from build123d import *

# Parameters (mm, degrees)
BOSS_EXTRUDE1_DEPTH = 12.7
SKETCH3_R           = 2.286
CUT_EXTRUDE1_DEPTH  = 232.948038146
CAVITY1_START       = -1
CAVITY1_OUTLINE_R   = 2.286
CAVITY1_DEPTH       = 15
CUT_EXTRUDE2_DEPTH  = 232.948038146
FILLET1_R           = 12.7
FILLET2_R           = 2.54
FILLET3_R           = 20.32
FILLET4_R           = 17.78
SKETCH5_W           = 16.51
SKETCH5_H           = 5.08
CUT_EXTRUDE3_DEPTH  = 230.304470216
FILLET5_R           = 127
FILLET6_R           = 50.8


with BuildPart() as part:
    # Sketch1 → Boss-Extrude1 (new body)
    with BuildSketch(Plane(origin=(0, 0, 0), x_dir=(1, 0, 0), z_dir=(0, 1, 0))):
        with BuildLine():
            Line((0, 0), (38.1, 0))
            Line((38.1, 0), (38.1, 25.4))
            ThreePointArc((38.1, 25.4), (19.393233119, 60.430202712), (-12.7, 83.82))
            Line((-12.7, 83.82), (-165.1, 83.82))
            ThreePointArc((-165.1, 83.82), (-197.193233119, 60.430202712), (-215.9, 25.4))
            Line((-215.9, 25.4), (-215.9, 0))
            Line((-215.9, 0), (-177.8, 0))
            ThreePointArc((-177.8, 0), (-166.58502935, 42.017514675), (-139.7, 76.2))
            Line((-139.7, 76.2), (-38.1, 76.2))
            ThreePointArc((-38.1, 76.2), (-11.21497065, 42.017514675), (0, 0))
        make_face()
    extrude(amount=BOSS_EXTRUDE1_DEPTH)

    # Sketch3 → Cut-Extrude1 (cut, through all)
    with BuildSketch(Plane(origin=(0, 12.7, 0), x_dir=(1, 0, 0), z_dir=(0, 1, 0))):
        with Locations(Location((19.05, 28.956, 0), (0, 0, 270))):
            Circle(SKETCH3_R)
    extrude(amount=-CUT_EXTRUDE1_DEPTH, mode=Mode.SUBTRACT)

    # Cavity1: read off the stored shape, not the designer's step
    # Cavity1 outline → Cavity1 (cut)
    with BuildSketch(Plane(origin=(0, 0, 0), x_dir=(1, 0, 0), z_dir=(0, 1, 0)).offset(CAVITY1_START)):
        with BuildLine():
            ThreePointArc((13.557199982, 23.797473427), (13.721594677, 23.627834729), (13.891225968, 23.463432392))
            ThreePointArc((13.891225968, 23.463432392), (15.144839416, 23.828362371), (16.075009031, 24.744607454))
            ThreePointArc((16.075009031, 24.744607454), (16.471799412, 24.490657889), (16.890111616, 24.273983275))
            ThreePointArc((16.890111616, 24.273983275), (16.561647975, 23.010325013), (16.872358933, 21.742184932))
            ThreePointArc((16.872358933, 21.742184932), (17.099548264, 21.677470858), (17.32865444, 21.619909903))
            ThreePointArc((17.32865444, 21.619909903), (18.231850543, 22.56275526), (18.579278518, 23.821331586))
            ThreePointArc((18.579278518, 23.821331586), (19.049883851, 23.799800001), (19.520490153, 23.821310384))
            ThreePointArc((19.520490153, 23.821310384), (19.867861426, 22.562718407), (20.77101505, 21.61983236))
            ThreePointArc((20.77101505, 21.61983236), (21.000123819, 21.677382993), (21.227316065, 21.742086832))
            ThreePointArc((21.227316065, 21.742086832), (21.538084156, 23.010212914), (21.209677446, 24.273885972))
            ThreePointArc((21.209677446, 24.273885972), (21.627999411, 24.490541739), (22.024801233, 24.744473428))
            ThreePointArc((22.024801233, 24.744473428), (22.954929568, 23.828186439), (24.208526573, 23.463199982))
            ThreePointArc((24.208526573, 23.463199982), (24.378165271, 23.627594677), (24.542567608, 23.797225968))
            ThreePointArc((24.542567608, 23.797225968), (24.177637629, 25.050839416), (23.261392546, 25.981009031))
            ThreePointArc((23.261392546, 25.981009031), (23.515342111, 26.377799412), (23.732016725, 26.796111616))
            ThreePointArc((23.732016725, 26.796111616), (24.995674987, 26.467647975), (26.263815068, 26.778358933))
            ThreePointArc((26.263815068, 26.778358933), (26.328529142, 27.005548264), (26.386090097, 27.23465444))
            ThreePointArc((26.386090097, 27.23465444), (25.44324474, 28.137850543), (24.184668414, 28.485278518))
            ThreePointArc((24.184668414, 28.485278518), (24.206199999, 28.955883851), (24.184689616, 29.426490153))
            ThreePointArc((24.184689616, 29.426490153), (25.443281593, 29.773861426), (26.38616764, 30.67701505))
            ThreePointArc((26.38616764, 30.67701505), (26.328617007, 30.906123819), (26.263913168, 31.133316065))
            ThreePointArc((26.263913168, 31.133316065), (24.995787086, 31.444084156), (23.732114028, 31.115677446))
            ThreePointArc((23.732114028, 31.115677446), (23.515458261, 31.533999411), (23.261526572, 31.930801233))
            ThreePointArc((23.261526572, 31.930801233), (24.177813561, 32.860929568), (24.542800018, 34.114526573))
            ThreePointArc((24.542800018, 34.114526573), (24.378405323, 34.284165271), (24.208774032, 34.448567608))
            ThreePointArc((24.208774032, 34.448567608), (22.955160584, 34.083637629), (22.024990969, 33.167392546))
            ThreePointArc((22.024990969, 33.167392546), (21.628200588, 33.421342111), (21.209888384, 33.638016725))
            ThreePointArc((21.209888384, 33.638016725), (21.538352025, 34.901674987), (21.227641067, 36.169815068))
            ThreePointArc((21.227641067, 36.169815068), (21.000451736, 36.234529142), (20.77134556, 36.292090097))
            ThreePointArc((20.77134556, 36.292090097), (19.868149457, 35.34924474), (19.520721482, 34.090668414))
            ThreePointArc((19.520721482, 34.090668414), (19.050116149, 34.112199999), (18.579509847, 34.090689616))
            ThreePointArc((18.579509847, 34.090689616), (18.232138574, 35.349281593), (17.32898495, 36.29216764))
            ThreePointArc((17.32898495, 36.29216764), (17.099876181, 36.234617007), (16.872683935, 36.169913168))
            ThreePointArc((16.872683935, 36.169913168), (16.561915844, 34.901787086), (16.890322554, 33.638114028))
            ThreePointArc((16.890322554, 33.638114028), (16.472000589, 33.421458261), (16.075198767, 33.167526572))
            ThreePointArc((16.075198767, 33.167526572), (15.145070432, 34.083813561), (13.891473427, 34.448800018))
            ThreePointArc((13.891473427, 34.448800018), (13.721834729, 34.284405323), (13.557432392, 34.114774032))
            ThreePointArc((13.557432392, 34.114774032), (13.922362371, 32.861160584), (14.838607454, 31.930990969))
            ThreePointArc((14.838607454, 31.930990969), (14.584657889, 31.534200588), (14.367983275, 31.115888384))
            ThreePointArc((14.367983275, 31.115888384), (13.104325013, 31.444352025), (11.836184932, 31.133641067))
            ThreePointArc((11.836184932, 31.133641067), (11.771470858, 30.906451736), (11.713909903, 30.67734556))
            ThreePointArc((11.713909903, 30.67734556), (12.65675526, 29.774149457), (13.915331586, 29.426721482))
            ThreePointArc((13.915331586, 29.426721482), (13.893800001, 28.956116149), (13.915310384, 28.485509847))
            ThreePointArc((13.915310384, 28.485509847), (12.656718407, 28.138138574), (11.71383236, 27.23498495))
            ThreePointArc((11.71383236, 27.23498495), (11.771382993, 27.005876181), (11.836086832, 26.778683935))
            ThreePointArc((11.836086832, 26.778683935), (13.104212914, 26.467915844), (14.367885972, 26.796322554))
            ThreePointArc((14.367885972, 26.796322554), (14.584541739, 26.378000589), (14.838473428, 25.981198767))
            ThreePointArc((14.838473428, 25.981198767), (13.922186439, 25.051070432), (13.557199982, 23.797473427))
        make_face()
        with Locations((19.05, 28.956)):
            Circle(CAVITY1_OUTLINE_R, mode=Mode.SUBTRACT)
    extrude(amount=CAVITY1_DEPTH, mode=Mode.SUBTRACT)

    # Sketch4 → Cut-Extrude2 (cut, through all)
    with BuildSketch(Plane(origin=(0, 12.7, 0), x_dir=(1, 0, 0), z_dir=(0, 1, 0))):
        with BuildLine():
            Line((38.1, 12.7), (-1.496322316, 12.7))
            ThreePointArc((-1.496322316, 12.7), (-0.559939387, 6.372176412), (0, 0))
            Line((0, 0), (38.1, 0))
            Line((38.1, 0), (38.1, 12.7))
        make_face()
    extrude(amount=-CUT_EXTRUDE2_DEPTH, mode=Mode.SUBTRACT)

    # Fillet1
    fillet1_edges = [part.edges().sort_by_distance(p)[0] for p in [
        (-1.496322316, 6.35, -12.7),
        (-177.8, 6.35, 0),
    ]]
    fillet(fillet1_edges, radius=FILLET1_R)

    # Fillet2
    fillet2_edges = [part.edges().sort_by_distance(p)[0] for p in [
        (-215.9, 6.35, 0),
    ]]
    fillet(fillet2_edges, radius=FILLET2_R)

    # Fillet3
    # the kernel refuses this fillet: 20.32 mm, written as the material it takes off along each edge
    with BuildSketch(Plane(origin=(38.1, 59.792860393, -12.7), x_dir=(0, 0, -1), z_dir=(0, -1, 0))) as fillet3_piece_1:
        with BuildLine():
            CenterArc((20.32, -18.837144157), FILLET3_R, 112.024312837, 67.975687163)
            Line((0, -18.837144157), (-0.4064, -18.837144157))
            Line((-0.4064, -18.837144157), (-0.4064, 0))
            Line((-0.4064, 0), (0, 0.4064))
            ThreePointArc((0, 0.4064), (6.35, 0.4064), (12.5476, 0.376742883))
            Line((12.5476, 0.376742883), (12.7, 0))
        make_face()
    extrude(amount=106.885720786, mode=Mode.SUBTRACT)

    # Fillet4
    fillet4_edges = [part.edges().sort_by_distance(p)[0] for p in [
        (38.1, 6.35, -25.4),
        (-139.7, 6.35, -76.2),
        (-38.1, 6.35, -76.2),
        (-12.7, 6.35, -83.82),
        (-165.1, 6.35, -83.82),
    ]]
    fillet(fillet4_edges, radius=FILLET4_R)

    # Sketch5 → Cut-Extrude3 (cut, through all)
    with BuildSketch(Plane.XY.offset(-76.2)):
        with Locations((-86.868, 0)):
            Rectangle(SKETCH5_W, SKETCH5_H)
    extrude(amount=-CUT_EXTRUDE3_DEPTH, mode=Mode.SUBTRACT)

    # Fillet5
    # the kernel refuses this fillet: 127 mm, written as the material it takes off along each edge
    with BuildSketch(Plane(origin=(-95.123, 0, -13.018297744), x_dir=(-1, 0, 0), z_dir=(0, 0, -1)), Plane(origin=(-78.613, 0, -147.001702256), x_dir=(1, 0, 0), z_dir=(0, 0, 1))) as fillet5_piece_1:
        with BuildLine():
            CenterArc((25.272680903, 127), FILLET5_R, 258.521659045, 11.478340955)
            Line((0, 2.54), (0, 0))
            Line((0, 0), (25.272680903, 0))
        make_face()
    extrude(amount=133.983404513, mode=Mode.SUBTRACT)

    # Fillet6
    fillet6_edges = [part.edges().sort_by_distance(p)[0] for p in [
        (-78.613, 2.54, -80.01),
        (-95.123, 2.54, -80.01),
    ]]
    fillet(fillet6_edges, radius=FILLET6_R)


solid = part.part
Could you check a few things on this model? Use its own coordinates, in mm. A direction names the side the tool comes from. Round coordinates to 2 decimals unless told otherwise and drop trailing zeros. Write each loop counter-clockwise with the first axis right and the second up, starting at its lowest first coordinate (ties: lowest second). Pieces come first, ordered by that corner, then holes. Notation, with made-up numbers: (56, 10.5) - (85, 10.5) arc R28 cw to (85, 31.5) - close; hole circle Ø11 at (67.25, -2). An arc over 180 degrees is marked (long way). Put each result on its own line as item: value. Start each with the question number.
(1) I want a section at A-A, the plane z = -48. Please give me the cut outline in (x, y), plus the area to 3 significant figures.
(2) For faces 5 (the cylindrical face through (0.85, 6.26, -15.38)), 6 (the cylindrical face through (-109.512, 0.467, -79.957)), 7 (the flat face through (-201, 6, 0)), 8 (the flat face through (13, 6, -12.7)), which set-ups out of +Z, -Z, +X, -X, +Y, -Y let a thin tool reach every point of the face, with its end or its side?
(3) Thinking about a two-plate mould opening in X: for faces 1 (the cylindrical face through (16.797, 6.261, -63.288)), 2 (the cylindrical face through (-78.933, 2.353, -80.063)), 3 (the flat face through (-100, 12.7, -82)), 4 (the cylindrical face through (-198.25, 6.26, -59.19)), which applies, released by +X, released by -X, zero draft, split by the parting line, or undercut?
(4) I want a section at C-C, the plane x = -130. Please give me the cut outline in (y, z), plus the area to 3 significant figures.
(5) I want a section at D-D, the plane x = -58. Please give me the cut outline in (y, z).
(6) I want a section at B-B, the plane z = -63.5. Please give me the cut outline in (x, y), plus the area to 3 significant figures.
(7) I need wall thicknesses on probe 1 along X at (y, z) = (5.75, -27); probe 2 along Z at (x, y) = (-76, 8.5); probe 3 along X at (y, z) = (8.5, -52). Which ranges of each line are inside material? Lowest first, please.
(8) Will these pins go through, and if not, where does the flat tip stop? pin 1 (2 mm diameter, centred on x = -86, z = -79, fed in from -Y); pin 2 (7 mm diameter, centred on x = 11.5, y = 8.5, fed in from +Z); pin 3 (4 mm diameter, centred on x = -89.5, y = 6.5, fed in from +Z).
Here are the results:
1. outline: (-206.24, 0) - (-163.35, 0) - (-163.35, 12.7) - (-206.24, 12.7) - close; (-14.45, 0) - (28.44, 0) - (28.44, 12.7) - (-14.45, 12.7) - close
1. area: 1,090 mm^2
2. face 5: +Z, +Y, -Y
2. face 6: +Z, -Z, -Y
2. face 7: +Z, +X, -X, +Y, -Y
2. face 8: +Z, +X, +Y, -Y
3. face 1: released by +X
3. face 2: undercut
3. face 3: zero draft
3. face 4: released by -X
4. outline: (0, -83.82) - (12.7, -83.82) - (12.7, -76.2) - (0, -76.2) - close
4. area: 96.8 mm^2
5. outline: (0.09, -83.82) - (12.7, -83.82) - (12.7, -76.2) - (0.09, -76.2) - close
6. outline: (-194.4, 0) - (-152.41, 0) - (-152.41, 12.7) - (-194.4, 12.7) - close; (-25.39, 0) - (16.6, 0) - (16.6, 12.7) - (-25.39, 12.7) - close
6. area: 1,070 mm^2
7. probe 1: x = -215.45 to -172.73, -5.07 to 11.77, 26.33 to 34.96
7. probe 2: z = -83.82 to -76.2
7. probe 3: x = -203.68 to -160.91, -16.89 to 25.88
8. pin 1: stops at y = 2.54
8. pin 2: stops at z = -12.7
8. pin 3: stops at z = -76.2
